Verification items for the finished model (mm, model axes). Coordinates: 2 decimals unless noted, no trailing zeros. Order: outer loops, then holes, each group sorted by start corner. A loop starts at its lowest first (then second) coordinate and runs counter-clockwise, first axis right, second up. Notation, with made-up numbers: (-22.75, 54.25) -> (1.25, 54.25) arc R24 ccw to (1.25, 69.25) -> close; hole circle Ø6 at (83, -36.5). An arc over 180 degrees is marked (long way). Write item = value, one per line. Start each with the question number.
1. Cross-section at C-C on z = 2.3. Record the cut outline in (x, y), plus the area to 3 significant figures.
2. Go/stop test with flat-tipped pins: P1, Ø2, axis at y = 2.5, z = -1.5, coming from the +X side; P2, Ø3.5, axis at x = 53, y = -1, coming from the -Z side. Record where each tip stops, or that it passes through.
3. Cross-section at B-B on y = 0. Record the cut outline in (x, z).
4. Cross-section at A-A on x = 24. Record the cut outline in (y, z), plus the area to 3 significant figures.
5. Thickness scan on line 1 along Y through (x, z) = (54, -0.75); line 2 along X through (y, z) = (2, -1.05); line 3 along Z through (x, y) = (-1, 0.25). Record the ranges inside material, lowest first. Write a range as from..to.
from build123d import *

# Parameters (mm, degrees)
BOSS_EXTRUDE1_DEPTH      = 3
BOSS_EXTRUDE1_DEPTH_BACK = 3
SKETCH1_R                = 2.2
BOSS_EXTRUDE2_START      = -2
SKETCH2_R                = 2.2
BOSS_EXTRUDE2_DEPTH      = 2
CHAMFER2_SIZE            = 1


with BuildPart() as part:
    # Sketch1 → Boss-Extrude1 (new, two sides: drawn at the far end of the back side and taken through both)
    with BuildSketch(Plane.XY.offset(-BOSS_EXTRUDE1_DEPTH_BACK)):
        with BuildLine():
            ThreePointArc((0, 4.5), (-4.5, 0), (0, -4.5))
            Line((0, -4.5), (54, -4.5))
            ThreePointArc((54, -4.5), (58.5, 0), (54, 4.5))
            Line((54, 4.5), (0, 4.5))
        make_face()
        Circle(SKETCH1_R, mode=Mode.SUBTRACT)
        with Locations((54, 0)):
            Circle(SKETCH1_R, mode=Mode.SUBTRACT)
    extrude(amount=BOSS_EXTRUDE1_DEPTH + BOSS_EXTRUDE1_DEPTH_BACK)

    # Sketch2 → Boss-Extrude2 (add)
    with BuildSketch(Plane.XY.offset(3).offset(BOSS_EXTRUDE2_START)):
        with Locations((54, 0)):
            Circle(SKETCH2_R)
        Circle(SKETCH2_R)
    extrude(amount=BOSS_EXTRUDE2_DEPTH)

    # Chamfer2
    chamfer2_edges = [part.edges().sort_by_distance(p)[0] for p in [
        (58.5, 0, -3),
        (27, 4.5, -3),
        (-4.5, 0, -3),
        (27, -4.5, -3),
    ]]
    chamfer(chamfer2_edges, length=CHAMFER2_SIZE)


solid = part.part
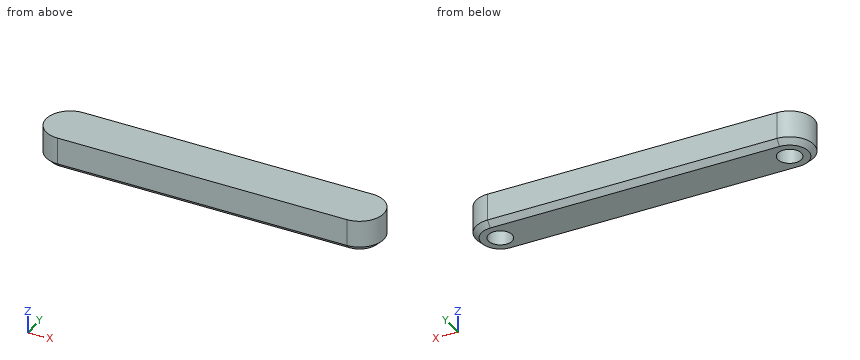
Worked out:
q1.outline = (0, -4.5) -> (54, -4.5) arc R4.5 ccw to (54, 4.5) -> (0, 4.5) arc R4.5 ccw to start
q1.area = 550 mm²
q2.P1 = 58.24
q2.P2 = -3
q3.outline = (-4.5, -2) -> (-3.5, -3) -> (-2.2, -3) -> (-2.2, 1) -> (2.2, 1) -> (2.2, -3) -> (51.8, -3) -> (51.8, 1) -> (56.2, 1) -> (56.2, -3) -> (57.5, -3) -> (58.5, -2) -> (58.5, 3) -> (-4.5, 3) -> close
q4.outline = (-4.5, -2) -> (-3.5, -3) -> (3.5, -3) -> (4.5, -2) -> (4.5, 3) -> (-4.5, 3) -> close
q4.area = 53.0 mm²
q5.line_1 = -4.5..-2.2, 2.2..4.5
q5.line_2 = -4.03..-0.92, 0.92..53.08, 54.92..58.03
q5.line_3 = 1..3
